from build123d import *

# Parameters (mm, degrees)
SKETCH_1_R        = 3.1
SKETCH_1_R_2      = 1.75
EXTRUDE_1_DEPTH   = 25
EXTRUDE_1_2_DEPTH = 25
SKETCH_2_R        = 1.75
EXTRUDE_2_DEPTH   = 2
SKETCH_3_W        = 30.176052102
SKETCH_3_H        = 2
EXTRUDE_3_DEPTH   = 15


with BuildPart() as part:
    # Sketch 1 → Extrude 1 (new body)
    with BuildSketch(Plane(origin=(0, 0, 0), x_dir=(1, 0, 0), z_dir=(0, 1, 0))):
        with Locations((-17.5, 0)):
            Circle(SKETCH_1_R)
        with Locations((-17.5, 0)):
            Circle(SKETCH_1_R_2, mode=Mode.SUBTRACT)
    extrude(amount=EXTRUDE_1_DEPTH)



with BuildPart() as body_2:
    # Sketch 1 → Extrude 1 2 (new body)
    with BuildSketch(Plane(origin=(0, 0, 0), x_dir=(1, 0, 0), z_dir=(0, 1, 0))):
        with Locations((17.5, 0)):
            Circle(SKETCH_1_R)
        with Locations((17.5, 0)):
            Circle(SKETCH_1_R_2, mode=Mode.SUBTRACT)
    extrude(amount=EXTRUDE_1_2_DEPTH)


with BuildPart() as part_1:
    add(part.part)

    add(body_2.part)  # Extrude 2 merges body 2
    # Sketch 2 → Extrude 2 (add)
    with BuildSketch(Plane.XZ):
        with BuildLine():
            Line((-17.5, 3.1), (17.5, 3.1))
            ThreePointArc((17.5, 3.1), (20.6, 0), (17.5, -3.1))
            Line((17.5, -3.1), (-17.5, -3.1))
            ThreePointArc((-17.5, -3.1), (-20.6, 0), (-17.5, 3.1))
        make_face()
        with Locations((-17.5, 0)):
            Circle(SKETCH_2_R, mode=Mode.SUBTRACT)
        with Locations((17.5, 0)):
            Circle(SKETCH_2_R, mode=Mode.SUBTRACT)
    extrude(amount=-EXTRUDE_2_DEPTH)

    # Sketch 3 → Extrude 3 (add)
    with BuildSketch(Plane(origin=(0, 2, 0), x_dir=(1, 0, 0), z_dir=(0, 1, 0))):
        Rectangle(SKETCH_3_W, SKETCH_3_H)
    extrude(amount=EXTRUDE_3_DEPTH)


solid = part_1.part
Design review of the part built by this model. Coordinates are the model's own, in mm. A direction names the side the tool comes from. Round coordinates to 2 decimals unless told otherwise and drop trailing zeros. Write each loop counter-clockwise with the first axis right and the second up, starting at its lowest first coordinate (ties: lowest second). Pieces come first, ordered by that corner, then holes. Notation, with made-up numbers: M -8.75,60 L 0.25,60 A8 cw 0.25,73 Z; hole C 22.25,11.25 d8. An arc over 180 degrees is marked long. One line per item, written item: value. Start each with the question number.
1. Take a section at D-D on y = 9. State the section outline as (x, z) points, then the cut area to 3 significant figures.
2. For faces 4 (the face through (0, 17, 0)), 5 (the face through (0, 9, 1)), 6 (the face through (0, 9, -1)), list the 3-axis set-ups (+Z, -Z, +X, -X, +Y, -Y) from which the entire face can be reached by the end or side of a thin tool; tool diameter is ignored.
3. Take a section at C-C on x = -1.5. State the section outline as (y, z) points.
4. Take a section at A-A on y = 20. State the section outline as (x, z) points, then the cut area to 3 significant figures.
5. To check wall thickness, follow probe 1 along X at (y, z) = (7.25, 0); probe 2 along X at (y, z) = (17.75, 0); probe 3 along Z at (x, y) = (-17.5, 11.75). State the ranges of each line that lie inside material, in increasing order. Write a range as from..to.
6. Take a section at B-B on z = 0. State the section outline as (x, y) points.
7. Draft analysis for pull direction Z (two halves, no side actions). For faces 1 (the face through (0, 0, 0)), 2 (the face through (0, 1, 3.1)), 3 (the face through (16.11, 12.32, 1.06)), state which applies: pulls with the +Z half, pulls with the -Z half, needs draft (parallel to the pull), parting line crosses it, or undercut.
8. Clearance check with flat-ended pins moving along their axes: P1, Ø1, axis at x = 0, z = 0, coming from the +Y side; P2, Ø3, axis at x = -17.5, z = 0, coming from the +Y side; P3, Ø2, axis at y = 17.5, z = 1.5, coming from the -X side; P4, Ø1.7, axis at x = -2.5, z = -2, coming from the +Y side. State where each tip first meets the part, or that it passes through.
Computed:
1. outline: M -14.57,-1 L 14.57,-1 A3.1 ccw long 14.57,1 L -14.57,1 A3.1 ccw long Z; hole C -17.5,0 d3.5; hole C 17.5,0 d3.5
1. area: 99.0 mm²
2. face 4: +Z, -Z, +Y
2. face 5: +Z, +Y
2. face 6: -Z, +Y
3. outline: M 0,-3.1 L 2,-3.1 L 2,-1 L 17,-1 L 17,1 L 2,1 L 2,3.1 L 0,3.1 Z
4. outline: C -17.5,0 d6.2; C 17.5,0 d6.2; hole C -17.5,0 d3.5; hole C 17.5,0 d3.5
4. area: 41.1 mm²
5. probe 1: x = -20.6..-19.25, -15.75..15.75, 19.25..20.6
5. probe 2: x = -20.6..-19.25, -15.75..-14.4, 14.4..15.75, 19.25..20.6
5. probe 3: z = -3.1..-1.75, 1.75..3.1
6. outline: M -20.6,0 L -19.25,0 L -19.25,25 L -20.6,25 Z; M -15.75,0 L 15.75,0 L 15.75,25 L 14.4,25 L 14.4,17 L -14.4,17 L -14.4,25 L -15.75,25 Z; M 19.25,0 L 20.6,0 L 20.6,25 L 19.25,25 Z
7. face 1: needs draft
7. face 2: pulls with the +Z half
7. face 3: undercut
8. P1: stops at y = 17
8. P2: passes through
8. P3: stops at x = -20.56
8. P4: stops at y = 2
